```python
from build123d import *

# Parameters (mm, degrees)
SCHIZZO1_R                        = 27
ESTRUSIONE_ESTRUSIONE1_DEPTH      = 1
SCHIZZO2_R                        = 8
TAGLIO_ESTRUSIONE1_DEPTH          = 39.19685851
SCHIZZO3_R                        = 27
SCHIZZO3_R_2                      = 13.6
ESTRUSIONE_ESTRUSIONE2_DEPTH      = 5
ESTRUSIONE_ESTRUSIONE3_DEPTH      = 2
ESTRUSIONE_ESTRUSIONE3_DEPTH_BACK = 1
SCHIZZO5_W                        = 65
SCHIZZO5_H                        = 42
SCHIZZO5_R                        = 13.6
TAGLIO_ESTRUSIONE2_START          = -27
TAGLIO_ESTRUSIONE2_OUTLINE_R      = 1.35
TAGLIO_ESTRUSIONE2_DEPTH          = 53.999999754
TAGLIO_ESTRUSIONE3_DEPTH          = 44.869308585
TAGLIO_ESTRUSIONE3_DEPTH_BACK     = 44.869308585
SCHIZZO8_W                        = 81.46070362
SCHIZZO8_H                        = 59.010327036
SCHIZZO8_W_2                      = 65
SCHIZZO8_H_2                      = 42
TAGLIO_ESTRUSIONE5_DEPTH          = 43.676105804
TAGLIO_ESTRUSIONE6_DEPTH          = 5
SCHIZZO13_R                       = 5
TAGLIO_ESTRUSIONE8_DEPTH          = 2
TAGLIO_ESTRUSIONE9_DEPTH          = 63.725779509
TAGLIO_ESTRUSIONE9_DEPTH_BACK     = 63.725779509
SCHIZZO3D3_R                      = 1.75


# Read off the part's stored shape, not the designer's step: Taglio-Estrusione2
with BuildPart() as part:
    # Schizzo1 → Estrusione-Estrusione1 (new body)
    with BuildSketch(Plane(origin=(0, 0, 0), x_dir=(1, 0, 0), z_dir=(0, 1, 0))):
        with Locations(Location((0, 0, 0), (0, 0, 270))):
            Circle(SCHIZZO1_R)
    extrude(amount=ESTRUSIONE_ESTRUSIONE1_DEPTH)

    # Schizzo2 → Taglio-Estrusione1 (cut, through all)
    with BuildSketch(Plane(origin=(0, 1, 0), x_dir=(1, 0, 0), z_dir=(0, 1, 0))):
        with Locations(Location((0, 0, 0), (0, 0, 270))):
            Circle(SCHIZZO2_R)
    extrude(amount=-TAGLIO_ESTRUSIONE1_DEPTH, mode=Mode.SUBTRACT)

    # Schizzo3 → Estrusione-Estrusione2 (add)
    with BuildSketch(Plane(origin=(0, 1, 0), x_dir=(1, 0, 0), z_dir=(0, 1, 0))):
        with Locations(Location((0, 0, 0), (0, 0, 270))):
            Circle(SCHIZZO3_R)
        with Locations(Location((0, 0, 0), (0, 0, 270))):
            Circle(SCHIZZO3_R_2, mode=Mode.SUBTRACT)
    extrude(amount=ESTRUSIONE_ESTRUSIONE2_DEPTH)

    # Schizzo5 → Estrusione-Estrusione3 (add, two sides: drawn at the far end of the back side and taken through both)
    with BuildSketch(Plane(origin=(0, 6, 0), x_dir=(1, 0, 0), z_dir=(0, 1, 0)).offset(-ESTRUSIONE_ESTRUSIONE3_DEPTH_BACK)):
        Rectangle(SCHIZZO5_W, SCHIZZO5_H)
        with Locations(Location((0, 0, 0), (0, 0, 270))):
            Circle(SCHIZZO5_R, mode=Mode.SUBTRACT)
    extrude(amount=ESTRUSIONE_ESTRUSIONE3_DEPTH + ESTRUSIONE_ESTRUSIONE3_DEPTH_BACK)

    # Taglio-Estrusione2 outline → Taglio-Estrusione2 (cut)
    with BuildSketch(Plane(origin=(0, 0, 0), x_dir=(0.866025403784438, 0, -0.500000000000001), z_dir=(0.500000000000001, 0, 0.866025403784438)).offset(TAGLIO_ESTRUSIONE2_START)):
        with Locations((0, 5)):
            Circle(TAGLIO_ESTRUSIONE2_OUTLINE_R)
    extrude(amount=TAGLIO_ESTRUSIONE2_DEPTH, mode=Mode.SUBTRACT)

    # Schizzo3D2 → Taglio-Estrusione3 (cut, two sides: drawn at the far end of the back side and taken through both)
    with BuildSketch(Plane(origin=(1.169134295, 5, -0.675), x_dir=(-0.41149103074101084, 0.8799053976571924, 0.23757445736745078), z_dir=(-0.5000000000000011, 1.0747888534457561e-14, -0.866025403784438)).offset(-TAGLIO_ESTRUSIONE3_DEPTH_BACK)):
        Polygon((0, 0), (1.28290207, -2.375744574), (5.682429058, 0), (4.399526988, 2.375744574), align=None)
    extrude(amount=TAGLIO_ESTRUSIONE3_DEPTH + TAGLIO_ESTRUSIONE3_DEPTH_BACK, mode=Mode.SUBTRACT)

    # Schizzo8 → Taglio-Estrusione5 (cut, through all)
    with BuildSketch(Plane(origin=(0, 6, 0), x_dir=(1, 0, 0), z_dir=(0, 1, 0))):
        Rectangle(SCHIZZO8_W, SCHIZZO8_H)
        Rectangle(SCHIZZO8_W_2, SCHIZZO8_H_2, mode=Mode.SUBTRACT)
    extrude(amount=-TAGLIO_ESTRUSIONE5_DEPTH, mode=Mode.SUBTRACT)

    # Schizzo9 → Taglio-Estrusione6 (cut)
    with BuildSketch(Plane.XZ):
        with BuildLine():
            Line((-22.997958605, -4.5), (-26.622359024, -4.5))
            Line((-26.622359024, -4.5), (-26.622359024, -10.5))
            Line((-26.622359024, -10.5), (-22.997958605, -10.5))
            ThreePointArc((-22.997958605, -10.5), (-19.997958605, -7.5), (-22.997958605, -4.5))
        make_face()
        with BuildLine():
            Line((22.997958605, 4.5), (27.800743069, 4.5))
            Line((27.800743069, 4.5), (27.800743069, 10.5))
            Line((27.800743069, 10.5), (22.997958605, 10.5))
            ThreePointArc((22.997958605, 10.5), (19.997958605, 7.5), (22.997958605, 4.5))
        make_face()
    extrude(amount=-TAGLIO_ESTRUSIONE6_DEPTH, mode=Mode.SUBTRACT)

    # Schizzo13 → Taglio-Estrusione8 (cut)
    with BuildSketch(Plane(origin=(0, 8, 0), x_dir=(1, 0, 0), z_dir=(0, 1, 0))):
        with Locations(Location((-22.997958605, 7.5, 0), (0, 0, 270))):
            Circle(SCHIZZO13_R)
        with Locations(Location((22.997958605, -7.5, 0), (0, 0, 270))):
            Circle(SCHIZZO13_R)
    extrude(amount=-TAGLIO_ESTRUSIONE8_DEPTH, mode=Mode.SUBTRACT)

    # Schizzo3D3 → Taglio-Estrusione9 (cut, two sides: drawn at the far end of the back side and taken through both)
    with BuildSketch(Plane(origin=(-22.997958605, 6.5, -7.5), x_dir=(0.9507217281959008, 0, 0.3100454733360893), z_dir=(0, -1, 0)).offset(-TAGLIO_ESTRUSIONE9_DEPTH_BACK)):
        with Locations(Location((0, 0, 0), (0, 0, 71.938029054))):
            Circle(SCHIZZO3D3_R)
        with Locations(Location((48.38, 0, 0), (0, 0, 71.938029054))):
            Circle(SCHIZZO3D3_R)
    extrude(amount=TAGLIO_ESTRUSIONE9_DEPTH + TAGLIO_ESTRUSIONE9_DEPTH_BACK, mode=Mode.SUBTRACT)


solid = part.part
```
For this review, take the finished solid that the model builds, in its own axes (mm). A direction names the side the tool comes from. Round coordinates to 2 decimals unless told otherwise and drop trailing zeros. Write each loop counter-clockwise with the first axis right and the second up, starting at its lowest first coordinate (ties: lowest second). Pieces come first, ordered by that corner, then holes. Notation, with made-up numbers: M -12,56 L 22,56 A32 cw 22,87 Z; hole C -30,72.5 d2. An arc over 180 degrees is marked long. One line per item, written item: value. Start each with the question number.
(1) Insertion check: pin 1 (0.9 mm diameter, centred on x = -23.5, y = 3.5, fed in from +Z); pin 2 (8 mm diameter, centred on x = -23, z = -8, fed in from +Y); pin 3 (3 mm diameter, centred on x = -23, z = -7.5, fed in from -Y); pin 4 (1.8 mm diameter, centred on x = 24.5, y = 3.5, fed in from +Z). Each pin has a flat end and moves straight along its axis. Give the tip position at first contact, or say it passes through.
(2) Wall thickness on line 1 (X direction, y = 0.5, z = 0); line 2 (Z direction, x = 0, y = 6.25); line 3 (Z direction, x = 10, y = 4.75): over which ranges is each line inside the solid? List them lowest first.
(3) We need section D-D (z = 0). Give the boundary of the cut face in (x, y).
(4) Machinability: for faces 4 (the flat face through (23, 6, 10)), 5 (the flat face through (25, 2, 4.5)), 6 (the cylindrical face through (-20, 2.5, -7.6)), 7 (the flat face through (0, 0, -10)), 8 (the flat face through (32.5, 6, 0)), which of the approach directions +Z, -Z, +X, -X, +Y, -Y give a long, thin tool a straight path to every point of the face, cutting with its end or side? Answer none if there is none.
(5) We need section A-A (y = 7). Give the boundary of the cut face in (x, z), and give its area (3 significant figures).
(6) The part is to be moulded in two halves that separate along X. For faces 1 (the cylindrical face through (21.515, 2.465, 16.312)), 2 (the flat face through (0, 5, -21)), 3 (the cylindrical face through (-24.18, 5.51, -8.79)), say which applies: released by +X, released by -X, zero draft, split by the parting line, or undercut.
(7) We need section B-B (x = 0). Give the boundary of the cut face in (y, z).
(8) We need section C-C (y = 2.5). Give the boundary of the cut face in (x, z).
Result:
1. pin 1: z = 14.06
1. pin 2: y = 6
1. pin 3: through
1. pin 4: z = 13.12
2. line 1: -27 to -8, 8 to 27
2. line 2: -21 to -13.6, 13.6 to 21
2. line 3: -21 to -9.22, 9.22 to 14.67, 19.97 to 21
3. outline: M -32.5,5 L -27,5 L -27,0 L -8,0 L -8,1 L -13.6,1 L -13.6,8 L -32.5,8 Z; M 8,0 L 27,0 L 27,5 L 32.5,5 L 32.5,8 L 13.6,8 L 13.6,1 L 8,1 Z
4. face 4: +Y
4. face 5: +X, -Y
4. face 6: -X, -Y
4. face 7: +Z, -Z, +X, -X, -Y
4. face 8: +Z, -Z, +X, +Y, -Y
5. outline: M -32.5,-21 L -13.68,-21 L -7.94,-11.04 A13.6 cw 5.6,12.39 L 10.57,21 L -32.5,21 Z; M -10.57,-21 L 32.5,-21 L 32.5,21 L 13.68,21 L 7.94,11.04 A13.6 cw -5.6,-12.39 Z; hole C -23,-7.5 d10; hole C 23,7.5 d10
5. area: 1,930 mm²
6. face 1: released by +X
6. face 2: zero draft
6. face 3: undercut
7. outline: M 0,-21 L 8,-21 L 8,-13.6 L 1,-13.6 L 1,-8 L 0,-8 Z; M 0,8 L 1,8 L 1,13.6 L 8,13.6 L 8,21 L 0,21 Z
8. outline: M -26.62,-4.5 L -23,-4.5 A3 cw -23,-10.5 L -24.87,-10.5 A27 ccw -16.97,-21 L 16.97,-21 A27 ccw 26.62,4.5 L 23,4.5 A3 cw 23,10.5 L 24.87,10.5 A27 ccw 16.97,21 L -16.97,21 A27 ccw Z; hole C 0,0 d27.2
